Design review of the part shown in the three views and the two pictorial views. Dimensions are in mm from the part's minimum x, y and z. Round coordinates to 2 decimals unless told otherwise and drop trailing zeros. Order: outer loops, then holes, each group sorted by start corner. A loop starts at its lowest first (then second) coordinate and runs counter-clockwise, first axis right, second up. Notation, with made-up numbers: (0, -8) - (57, -8) arc R25 cw to (57, 24) - close; hole circle Ø2 at (63.25, 33.5). An arc over 180 degrees is marked (long way). One line per item, written item: value.
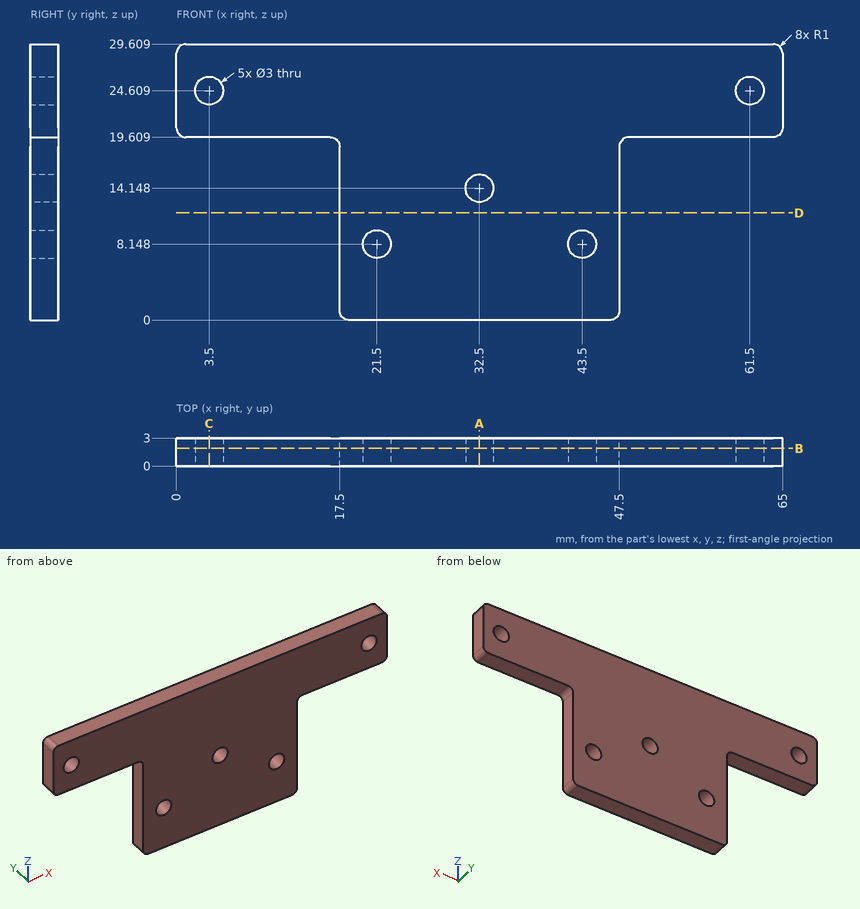
Item 1: Take a section at C-C (x = 3.5). Write out the cut boundary in (y, z).
Returned:
outline: (0, 19.61) - (3, 19.61) - (3, 23.11) - (0, 23.11) - close; (0, 26.11) - (3, 26.11) - (3, 29.61) - (0, 29.61) - close
Item 2: For P1, Ø1.8, axis at x = 21.5, z = 8.15, coming from the -Y side; P2, Ø1.5, axis at x = 6.5, y = 1.5, coming from the -Z side; P3, Ø1, axis at y = 2.5, z = 20, coming from the -X side; P4, Ø0.9, axis at y = 1, z = 6.5, coming from the +X side, all flat-tipped, find the tip position at first contact; note any pin that passes through.
Returned:
P1: through
P2: z = 19.61
P3: x = 0.01
P4: x = 47.5
Item 3: Wall thickness on line 1 (X direction, y = 2.35, z = 8); line 2 (Z direction, x = 43.5, y = 2.15); line 3 (X direction, y = 2.85, z = 7.25): over which ranges is each line inside the solid? List them lowest first.
Returned:
line 1: 17.5 to 20.01, 22.99 to 42.01, 44.99 to 47.5
line 2: 0 to 6.65, 9.65 to 29.61
line 3: 17.5 to 20.3, 22.7 to 42.3, 44.7 to 47.5
Item 4: Take a section at B-B (y = 1.9). Write out the cut boundary in (x, z), plus the area to 3 significant figures.
Returned:
outline: (0, 20.61) arc R1 ccw to (1, 19.61) - (16.5, 19.61) arc R1 cw to (17.5, 18.61) - (17.5, 1) arc R1 ccw to (18.5, 0) - (46.5, 0) arc R1 ccw to (47.5, 1) - (47.5, 18.61) arc R1 cw to (48.5, 19.61) - (64, 19.61) arc R1 ccw to (65, 20.61) - (65, 28.61) arc R1 ccw to (64, 29.61) - (1, 29.61) arc R1 ccw to (0, 28.61) - close; hole circle Ø3 at (3.5, 24.61); hole circle Ø3 at (21.5, 8.15); hole circle Ø3 at (32.5, 14.15); hole circle Ø3 at (43.5, 8.15); hole circle Ø3 at (61.5, 24.61)
area: 1,200 mm^2
Item 5: Take a section at A-A (x = 32.5). Write out the cut boundary in (y, z).
Returned:
outline: (0, 0) - (3, 0) - (3, 12.65) - (0, 12.65) - close; (0, 15.65) - (3, 15.65) - (3, 29.61) - (0, 29.61) - close
Item 6: Take a section at D-D (z = 11.5). Write out the cut boundary in (x, y).
Returned:
outline: (17.5, 0) - (47.5, 0) - (47.5, 3) - (17.5, 3) - close
